Check sheet for the drawn part. Datum: minimum x, y, z corner. Units: mm. A direction names the side the tool comes from. Coordinates: 2 decimals unless noted, no trailing zeros. Loops run counter-clockwise (first coordinate to the right, second up) from the corner with the lowest first, then second, coordinate; pieces in that order, holes last. Notation, with made-up numbers: (73, 7) -> (112, 7) arc R8 ccw to (112, 14) -> close; hole circle Ø1 at (6.5, -37). An arc over 180 degrees is marked (long way). Use CSV: the item, a comma, the result in double quotes. Start each with the question number.
1. Gauge pin test, flat ends, axial feed: pin 1 (12 mm diameter, centred on x = 6.5, y = 4.5, fed in from +Z); pin 2 (3 mm diameter, centred on x = 20, z = 47.32, fed in from -Y); pin 3 (2 mm diameter, centred on y = 8.5, z = 42.5, fed in from -X); pin 4 (4.5 mm diameter, centred on x = 20, z = 30, fed in from +Y). Record the tip position at first contact, or that the pin passes through.
2. Sectioned sample at B-B, the plane z = 26.5. Record the cut outline in (x, y) (1 decimal), and give its area (3 significant figures).
3. Thickness scan on L1, parallel to Z at x = 20, y = 3.25 (1 decimal); L2, parallel to Z at x = 35, y = 18.5; L3, parallel to X at y = 21.75, z = 30. Record the ranges inside material, lowest first.
4. Sectioned sample at C-C, the plane y = 19. Record the cut outline in (x, z), and give its area (3 significant figures).
5. Set-up check for the marked faces 1 and 2: record each of +Z, -Z, +X, -X, +Y, -Y from which the full face is reachable in a straight line by a thin tool's end or side.
6. Sectioned sample at D-D, the plane z = 8. Record the cut outline in (x, y), and give its area (3 significant figures).
7. Sectioned sample at A-A, the plane x = 30. Record the cut outline in (y, z).
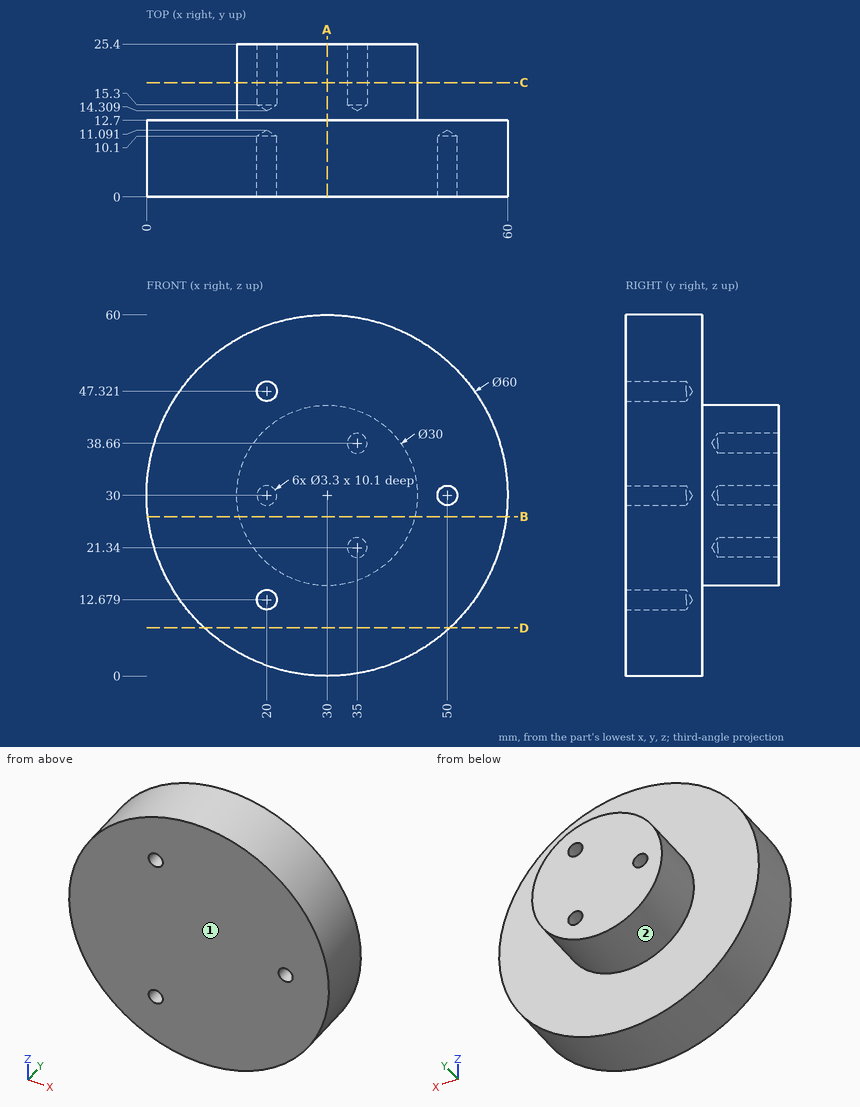
Completed:
1,pin 1,"z = 54.37"
1,pin 2,"y = 10.19"
1,pin 3,"x = 2.29"
1,pin 4,"y = 25.4"
2,outline,"(0.2, 0) -> (59.8, 0) -> (59.8, 12.7) -> (44.6, 12.7) -> (44.6, 25.4) -> (15.4, 25.4) -> (15.4, 12.7) -> (0.2, 12.7) -> close"
2,area,"1,130 mm²"
3,L1,"1.7 to 11, 14.3 to 45.7, 49 to 58.3"
3,L2,"15.86 to 19.69, 22.99 to 37.01, 40.31 to 44.14"
3,L3,"15 to 18.35, 21.65 to 45"
4,outline,"circle Ø30 at (30, 30); hole circle Ø3.3 at (20, 30); hole circle Ø3.3 at (35, 21.34); hole circle Ø3.3 at (35, 38.66)"
4,area,"681 mm²"
5,face 1,"+Z, -Z, +X, -X, -Y"
5,face 2,"+Y"
6,outline,"(9.6, 0) -> (50.4, 0) -> (50.4, 12.7) -> (9.6, 12.7) -> close"
6,area,"518 mm²"
7,outline,"(0, 0) -> (12.7, 0) -> (12.7, 15) -> (25.4, 15) -> (25.4, 45) -> (12.7, 45) -> (12.7, 60) -> (0, 60) -> close"
